Can you work these out from the model? Positions are in its coordinate system, mm. A direction names the side the tool comes from. Round coordinates to 2 decimals unless told otherwise and drop trailing zeros. Order: outer loops, then holes, each group sorted by start corner. A loop starts at its lowest first (then second) coordinate and runs counter-clockwise, first axis right, second up. Notation, with made-up numbers: M -27,44 L -3,44 A25 ccw -3,61 Z; hole C 7.5,35 d1. An arc over 180 degrees is marked long. Answer as a JSON object with one key per item and string values. Group by question number.
```python
from build123d import *

# Parameters (mm, degrees)
F0_W     = 25.4
F0_H     = 19.05
F1_DEPTH = 25.4
F2_T     = -2.54
F3_R     = 3.81
F5_DEPTH = 25.4
F4_R     = 3.81
F6_DEPTH = 25.4


with BuildPart() as f1:
    # F0 (on Front) → F1 (new body)
    with BuildSketch(Plane.XZ):
        Rectangle(F0_W, F0_H)
    extrude(amount=F1_DEPTH)

    # F2
    f2_openings = [f1.faces().sort_by_distance(p)[0] for p in [
        (12.7, -12.7, 0),
        (0, -12.7, 9.525),
        (0, 0, 0),
        (-12.7, -12.7, 0),
    ]]
    offset(amount=F2_T, openings=f2_openings)

    # F3 (on face) → F5 (cut)
    with BuildSketch(Plane(origin=(0, -22.86, 0), x_dir=(-1, 0, 0), z_dir=(0, 1, 0))):
        Circle(F3_R)
    extrude(amount=-F5_DEPTH, mode=Mode.SUBTRACT)

    # F4 (on face) → F6 (cut)
    with BuildSketch(Plane.XY.offset(-6.985)):
        with Locations((0, -12.414872)):
            Circle(F4_R)
    extrude(amount=-F6_DEPTH, mode=Mode.SUBTRACT)


solid = f1.part
```
1) For pin 1 (7 mm diameter, centred on x = 1.5, y = -11, fed in from +Z) (3 decimals); pin 2 (10 mm diameter, centred on x = 2, z = 3.5, fed in from +Y), each with a flat end and sliding along its axis, tell me the tip position at first contact or that it passes through.
2) Which directions (+Z, -Z, +X, -X, +Y, -Y) give clear straight access to the entire face, cutting with the end or side of a thin tool? Please do faces 4 (the face through (0, -24, 9.525)), 5 (the face through (3, -22.86, 3)).
3) If we section it at D-D on y = -18.75: Write out the boundary of the cut face in (x, z) (3 decimals).
4) If we section it at A-A on z = 0: Write out the boundary of the cut face in (x, y).
5) We'd pull the mould along X, two halves only. Please class faces 1 (the face through (-0.496, -8.637, -8.237)), 2 (the face through (-12.7, -16, -8)), 3 (the face through (3, -9, -6.985)): +X half, -X half, draft (parallel to the pull), parting line (faces both ways), or undercut.
6) If we section it at C-C on x = -6.75: Write out the boundary of the cut face in (y, z) (3 decimals).
7) If we section it at B-B on x = 0: Write out the boundary of the cut face in (y, z) (3 decimals).
8) I need wall thicknesses on line 1 along Y through (x, z) = (0, -7.75); line 2 along Z through (x, y) = (0.25, -18.25) (3 decimals); line 3 along Y through (x, z) = (5.75, 5.75). Which ranges of each line are inside material? Lowest first, please.
Findings:
{
 "1": {"pin 1": "stops at z = -6.985", "pin 2": "stops at y = -22.86"},
 "2": {"face 4": "+Z, +X, -X, +Y, -Y", "face 5": "+Z, +X, -X, +Y"},
 "3": {"outline": "M -12.7,-9.525 L 12.7,-9.525 L 12.7,-6.985 L -12.7,-6.985 Z"},
 "4": {"outline": "M -12.7,-25.4 L -3.81,-25.4 L -3.81,-22.86 L -12.7,-22.86 Z; M 3.81,-25.4 L 12.7,-25.4 L 12.7,-22.86 L 3.81,-22.86 Z"},
 "5": {"face 1": "undercut", "face 2": "-X half", "face 3": "draft"},
 "6": {"outline": "M -25.4,-9.525 L 0,-9.525 L 0,-6.985 L -22.86,-6.985 L -22.86,9.525 L -25.4,9.525 Z"},
 "7": {"outline": "M -25.4,-9.525 L -16.225,-9.525 L -16.225,-6.985 L -22.86,-6.985 L -22.86,-3.81 L -25.4,-3.81 Z; M -25.4,3.81 L -22.86,3.81 L -22.86,9.525 L -25.4,9.525 Z; M -8.605,-9.525 L 0,-9.525 L 0,-6.985 L -8.605,-6.985 Z"},
 "8": {"line 1": "y = -25.4 to -16.22, -8.6 to 0", "line 2": "z = -9.525 to -6.985", "line 3": "y = -25.4 to -22.86"}
}
